```python
from build123d import *

# Parameters (mm, degrees)
F0_W      = 42
F0_H      = 17
F1_DEPTH  = 7
F4_DEPTH  = 25
F5_W      = 42
F5_H      = 5.2
F6_DEPTH  = 10
F7_R      = 1.675
F8_DEPTH  = 25
F9_DEPTH  = 25
F10_W     = 5.7
F10_H     = 7
F11_DEPTH = 5


with BuildPart() as f1:
    # F0 (on Top) → F1 (new body)
    with BuildSketch(Plane.XY):
        with Locations((21, 8.5)):
            Rectangle(F0_W, F0_H)
    extrude(amount=F1_DEPTH)

    # F3 (on face) → F4 (cut)
    with BuildSketch(Plane(origin=(0, 17, 0), x_dir=(-1, 0, 0), z_dir=(0, 1, 0))):
        with BuildLine():
            ThreePointArc((-26.5, 3.5), (-25, 2), (-23.5, 3.5))
            ThreePointArc((-23.5, 3.5), (-25, 5), (-26.5, 3.5))
        make_face()
    extrude(amount=-F4_DEPTH, mode=Mode.SUBTRACT)

    # F5 (on face) → F6 (join)
    with BuildSketch(Plane.XY.offset(7)):
        with Locations((21, 14.4)):
            Rectangle(F5_W, F5_H)
    extrude(amount=F6_DEPTH)

    # F7 (on face) → F8 (cut)
    with BuildSketch(Plane(origin=(0, 17, 0), x_dir=(-1, 0, 0), z_dir=(0, 1, 0))):
        with Locations((-36.5, 12.325)):
            Circle(F7_R)
        with Locations((-5.5, 12.325)):
            Circle(F7_R)
    extrude(amount=-F8_DEPTH, mode=Mode.SUBTRACT)

    # F2 (on face) → F9 (cut)
    with BuildSketch(Plane.XY.offset(7)):
        with BuildLine():
            ThreePointArc((18.9686269666, 4.5), (18.9921490369, 4.7495083498), (19, 5))
            ThreePointArc((19, 5), (18.9921490369, 5.2504916502), (18.9686269666, 5.5))
            ThreePointArc((18.9686269666, 5.5), (11, 5), (18.9686269666, 4.5))
        make_face()
        with BuildLine():
            Line((42, 5), (19, 5))
            ThreePointArc((19, 5), (18.9921490369, 4.7495083498), (18.9686269666, 4.5))
            Line((18.9686269666, 4.5), (42, 4.5))
            Line((42, 4.5), (42, 5))
        make_face()
        with BuildLine():
            ThreePointArc((18.9686269666, 5.5), (18.9921490369, 5.2504916502), (19, 5))
            Line((19, 5), (42, 5))
            Line((42, 5), (42, 5.5))
            Line((42, 5.5), (18.9686269666, 5.5))
        make_face()
    extrude(amount=-F9_DEPTH, mode=Mode.SUBTRACT)

    # F10 (on face) → F11 (join)
    with BuildSketch(Plane(origin=(0, 0, 0), x_dir=(0, -1, 0), z_dir=(-1, 0, 0))):
        with Locations((-9.45, 3.5)):
            Rectangle(F10_W, F10_H)
    extrude(amount=F11_DEPTH)


solid = f1.part
```
For this review, take the finished solid that the model builds, in its own axes (mm). A direction names the side the tool comes from. Round coordinates to 2 decimals unless told otherwise and drop trailing zeros. Write each loop counter-clockwise with the first axis right and the second up, starting at its lowest first coordinate (ties: lowest second). Pieces come first, ordered by that corner, then holes.
1) Take a section at C-C on x = 36.5. Give the boundary of the cut face in (y, z), then the cut area to 3 significant figures.
Answer below:
outline: (0, 0) - (4.5, 0) - (4.5, 7) - (0, 7) - close; (5.5, 0) - (17, 0) - (17, 10.65) - (11.8, 10.65) - (11.8, 7) - (5.5, 7) - close; (11.8, 14) - (17, 14) - (17, 17) - (11.8, 17) - close
area: 147 mm2
2) Mouldability with a two-part tool opening along X and no side actions: class faces 6 (the face through (5.9, 14.4, 10.7)), 7 (the face through (42, 12, 6)), 8 (the face through (-2, 12.3, 3)) as +X half, -X half, draft (parallel to the pull), parting line (faces both ways), or undercut.
Answer below:
face 6: undercut
face 7: +X half
face 8: draft
3) Insertion check: pin 1 Ø1.6 at (y, z) = (14.5, 7.5) entering from -X; pin 2 Ø3 at (x, z) = (16, 10.5) entering from -Y; pin 3 Ø4 at (x, z) = (-3, 5) entering from +Y; pin 4 Ø2.5 at (x, z) = (25, 3.5) entering from +Y. Each pin has a flat end and moves straight along its axis. Give the tip position at first contact, or say it passes through.
Answer below:
pin 1: stops at x = 0
pin 2: stops at y = 11.8
pin 3: stops at y = 12.3
pin 4: passes through
4) Take a section at B-B on y = 1.5. Give the boundary of the cut face in (x, z), then the cut area to 3 significant figures.
Answer below:
outline: (0, 0) - (13.06, 0) - (13.06, 7) - (0, 7) - close; (16.94, 0) - (42, 0) - (42, 7) - (16.94, 7) - close; hole circle Ø3 at (25, 3.5)
area: 260 mm2
5) Machinability: for faces 1 (the face through (31, 5.5, 4)), 2 (the face through (-2, 6.6, 3)), 3 (the face through (21, 11.8, 12)), 4 (the face through (21, 14, 17)), 5 (the face through (26.5, 2.28, 3.57)), which of the approach directions +Z, -Z, +X, -X, +Y, -Y give a long, thin tool a straight path to every point of the face, cutting with its end or side? Answer none if there is none.
Answer below:
face 1: +Z, -Z, +X
face 2: +Z, -Z, -X, -Y
face 3: +Z, +X, -X, -Y
face 4: +Z, +X, -X, +Y, -Y
face 5: +Y, -Y
6) Take a section at A-A on x = 25. Give the boundary of the cut face in (y, z), then the cut area to 3 significant figures.
Answer below:
outline: (0, 0) - (4.5, 0) - (4.5, 2) - (0, 2) - close; (0, 5) - (4.5, 5) - (4.5, 7) - (0, 7) - close; (5.5, 0) - (17, 0) - (17, 2) - (5.5, 2) - close; (5.5, 5) - (17, 5) - (17, 17) - (11.8, 17) - (11.8, 7) - (5.5, 7) - close
area: 116 mm2
7) For line 1 along Y through (x, z) = (33.5, 1.25); line 2 along Z through (x, y) = (25, 2.4); line 3 along Y through (x, z) = (15, 2.25), list the stretches that pass through material, from the lowest coordinate up.
Answer below:
line 1: y = 0 to 4.5, 5.5 to 17
line 2: z = 0 to 2, 5 to 7
line 3: y = 0 to 1, 9 to 17
8) Take a section at D-D on x = 5.5. Give the boundary of the cut face in (y, z).
Answer below:
outline: (0, 0) - (17, 0) - (17, 10.65) - (11.8, 10.65) - (11.8, 7) - (0, 7) - close; (11.8, 14) - (17, 14) - (17, 17) - (11.8, 17) - close
